Input: part model. Units: mm. Frame: model coordinates. A direction names the side the tool comes from. Give positions to 0.01 mm unless a question says otherwise; leave off trailing zeros. Loops run counter-clockwise (first coordinate to the right, second up) from the corner with the lowest first, then second, coordinate; pieces in that order, holes last.
from build123d import *

# Parameters (mm, degrees)
F0_W     = 50
F0_H     = 50
F1_DEPTH = 900
F2_W     = 1250
F2_H     = 1250
F3_DEPTH = 40


with BuildPart() as f1:
    # F0 (on Top) → F1 (new body)
    with BuildSketch(Plane.XY):
        with Locations((-575, 575)):
            Rectangle(F0_W, F0_H)
        with Locations((575, 575)):
            Rectangle(F0_W, F0_H)
        with Locations((575, -575)):
            Rectangle(F0_W, F0_H)
        with Locations((-575, -575)):
            Rectangle(F0_W, F0_H)
    extrude(amount=F1_DEPTH)

    # F2 (on face) → F3 (join)
    with BuildSketch(Plane.XY.offset(900)):
        Rectangle(F2_W, F2_H)
    extrude(amount=F3_DEPTH)


solid = f1.part
(1) Cut plane B-B (x = -499.5). Return the cut outline in (y, z), and give its area (3 significant figures).
Values follow:
outline: (-625, 900) - (625, 900) - (625, 940) - (-625, 940) - close
area: 50,000 mm2
(2) Mould query, pull axis Y, two halves, no side actions, for faces 6 (the flat face through (625, -9, 920)), 7 (the flat face through (575, -600, 444)), 8 (the flat face through (-575, -550, 444)). Classes: +Y half, -Y half, draft (parallel to the pull), parting line (faces both ways), or undercut.
Values follow:
face 6: draft
face 7: -Y half
face 8: undercut
(3) Reachability of faces 1 (the flat face through (-550, 575, 444)), 2 (the flat face through (-575, 550, 444)), 3 (the flat face through (600, 575, 444)), 4 (the flat face through (-600, -575, 444)), 5 (the flat face through (-575, 600, 444)) from +Z, -Z, +X, -X, +Y, -Y: full face, straight path, thin tool, end or side. Return the list, or none.
Values follow:
face 1: -Z, +Y, -Y
face 2: -Z, +X, -X
face 3: -Z, +X, +Y, -Y
face 4: -Z, -X, +Y, -Y
face 5: -Z, +X, -X, +Y
(4) Pin query (flat end, axial travel): pin 1 Ø25 at (y, z) = (568.5, 508) entering from -X; pin 2 Ø25 at (x, z) = (-576.5, 660.5) entering from +Y; pin 3 Ø25 at (y, z) = (-582, 541.5) entering from +X. Return the tip coordinate at first contact, or that it passes through.
Values follow:
pin 1: stops at x = -600
pin 2: stops at y = 600
pin 3: stops at x = 600
(5) Cut plane A-A (z = 251.5). Return the cut outline in (x, y).
Values follow:
outline: (-600, -600) - (-550, -600) - (-550, -550) - (-600, -550) - close; (-600, 550) - (-550, 550) - (-550, 600) - (-600, 600) - close; (550, -600) - (600, -600) - (600, -550) - (550, -550) - close; (550, 550) - (600, 550) - (600, 600) - (550, 600) - close
(6) Ray query, probe 1 along X at (y, z) = (566, 713.5); probe 2 along Z at (x, y) = (188, -190.5). Return the intervals inside material, ascending.
Values follow:
probe 1: x = -600 to -550, 550 to 600
probe 2: z = 900 to 940
